Answer from the drawing. Dimensions are ordinates in mm from the lowest x, y and z of the part. Round coordinates to 2 decimals unless told otherwise and drop trailing zeros. Loops run counter-clockwise (first coordinate to the right, second up) from the corner with the lowest first, then second, coordinate; pieces in that order, holes last. Notation, with made-up numbers: M -40,84.25 L 11,84.25 A27 cw 11,113.25 Z; hole C -9,30.5 d2. An arc over 180 degrees is marked long. Write each question's results on one line, items separated by ' | '.
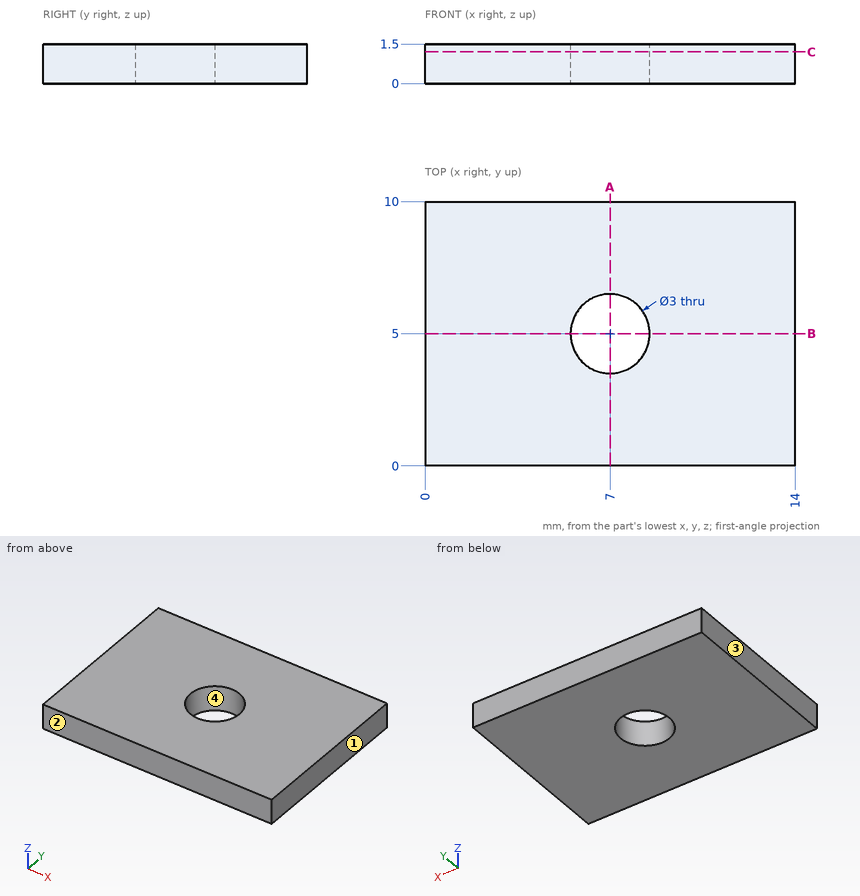
1. Determine the mould class of the marked faces 1, 2, 3 and 4 for opening direction X: released by +X, released by -X, zero draft, split by the parting line, or undercut.
Completed:
face 1: released by +X | face 2: zero draft | face 3: released by -X | face 4: undercut
2. Find the intervals of material crossed by L1, parallel to Y at x = 7, z = 0.6; L2, parallel to Y at x = 5.75, z = 1; L3, parallel to X at y = 5.5, z = 0.45, in increasing order.
Completed:
L1: y = 0 to 3.5, 6.5 to 10 | L2: y = 0 to 4.17, 5.83 to 10 | L3: x = 0 to 5.59, 8.41 to 14
3. Find section C-C, the plane z = 1.2. Give the vertices of the cut face in (x, y).
Completed:
outline: M 0,0 L 14,0 L 14,10 L 0,10 Z; hole C 7,5 d3
4. Find section A-A, the plane x = 7. Give the vertices of the cut face in (y, z), then the cut area to 3 significant figures.
Completed:
outline: M 0,0 L 3.5,0 L 3.5,1.5 L 0,1.5 Z; M 6.5,0 L 10,0 L 10,1.5 L 6.5,1.5 Z | area: 10.5 mm2
5. Find section B-B, the plane y = 5. Give the vertices of the cut face in (x, z).
Completed:
outline: M 0,0 L 5.5,0 L 5.5,1.5 L 0,1.5 Z; M 8.5,0 L 14,0 L 14,1.5 L 8.5,1.5 Z
